Autodesk Inventor part; units mm, degrees
ref_plane "YZ Plane" through (0, 0, 0) normal (1, 0, 0) x (0, 1, 0)
ref_plane "XZ Plane" through (0, 0, 0) normal (0, 1, 0) x (-1, 0, 0)
ref_plane "XY Plane" through (0, 0, 0) normal (0, 0, 1) x (1, 0, 0)
sketch "Sketch1" plane through (0, 0, 0) normal (0, 0, 1) x (1, 0, 0)
  line L0 (0, 0) -> (33.25, 0)
  line L1 (33.25, 0) -> (33.25, 33.25)
  line L2 (33.25, 33.25) -> (0, 33.25)
  line L3 (0, 33.25) -> (0, 0)
  dimension "d0" = 33.25
  dimension "d1" = 33.25
extrude "Extrusion1" add sketch "Sketch1" along normal blind 30
sketch "Sketch2" plane through (0, 0, 30) normal (0, 0, 1) x (1, 0, 0)
  point P0 (0, 0)
sketch "Sketch3" plane through (0, 0, 30) normal (0, 0, 1) x (1, 0, 0)
  line L0 (3.25, 3.25) -> (30, 3.25)
  line L1 (30, 3.25) -> (30, 30)
  line L2 (30, 30) -> (3.25, 30)
  line L3 (3.25, 30) -> (3.25, 3.25)
  line L4 (33.25, 0) -> (33.25, 33.25)
  line L5 (0, 0) -> (33.25, 0)
  line L6 (33.25, 0) -> (33.25, 33.25)
  line L7 (33.25, 33.25) -> (0, 33.25)
  line L8 (0, 33.25) -> (0, 0)
  dimension "d4" = 26.75
  dimension "d5" = 26.75
extrude "Extrusion2" cut sketch "Sketch3" against normal blind 26.75 contours L3 L2 L1 L0
chamfer "Chamfer1" distance 1.875 angle 45 8 edges at (33.25, 33.25, 15) (33.25, 0, 15) (0, 33.25, 15) (0, 0, 15) (0, 16.625, 0) (16.625, 33.25, 0) (16.625, 0, 0) (33.25, 16.625, 0)
sketch "Sketch4" plane through (0, 0, 0) normal (0, 0, -1) x (-1, 0, 0)
  circle A0 centre (-16.625, 16.625) radius 4.625
  point P0 (0, 0)
  dimension "d11" = 9.25
properties part number "cuvette holder lid"
Could you check a few things on this model? Use its own coordinates, in mm. A direction names the side the tool comes from. Coordinates: 2 decimals unless noted, no trailing zeros. Write each loop counter-clockwise with the first axis right and the second up, starting at its lowest first coordinate (ties: lowest second). Pieces come first, ordered by that corner, then holes. Notation, with made-up numbers: (66.25, -19) - (108.25, -19) arc R20 cw to (108.25, 8) - close; hole circle Ø6 at (73.25, 59.5). An arc over 180 degrees is marked (long way). Put each result on its own line as item: value. Start each with the question number.
Q1. I want a section at A-A on z = 7.5. Write out the boundary of the cut face in (x, y) (3 decimals).
Q2. Thinking about a two-plate mould opening in X: for faces 3 (the flat face through (3.25, 17, 17)), 4 (the flat face through (16, 17, 0)), 5 (the flat face through (0.951, 32.326, 15.741)), which applies, pulls with the +X half, pulls with the -X half, needs draft (parallel to the pull), parting line crosses it, or undercut?
Q3. Please list where these lines run through material, in increasing order: L1, parallel to Y at x = 19, z = 4.25; L2, parallel to Z at x = 10.5, y = 16.
Q4. I want a section at B-B on x = 19.5. Write out the boundary of the cut face in (y, z) (3 decimals).
Q5. Which directions (+Z, -Z, +X, -X, +Y, -Y) give clear straight access to the entire face, cutting with the end or side of a thin tool? Please do faces 1 (the flat face through (2, 17, 30)), 2 (the flat face through (16, 17, 3.25)).
Q6. I'm going to push a flat-ended pin straight in: P1, Ø8, axis at x = 20.5, y = 12.5, coming from the +Z side. Where does the tip first touch, or does it pass through?
Checks:
1. outline: (0, 1.875) - (1.875, 0) - (31.375, 0) - (33.25, 1.875) - (33.25, 31.375) - (31.375, 33.25) - (1.875, 33.25) - (0, 31.375) - close; hole (3.25, 3.25) - (30, 3.25) - (30, 30) - (3.25, 30) - close
2. face 3: undercut
2. face 4: needs draft
2. face 5: pulls with the -X half
3. L1: 0 to 3.25, 30 to 33.25
3. L2: 0 to 3.25
4. outline: (0, 1.875) - (1.875, 0) - (31.375, 0) - (33.25, 1.875) - (33.25, 30) - (30, 30) - (30, 3.25) - (3.25, 3.25) - (3.25, 30) - (0, 30) - close
5. face 1: +Z, +X, -X, +Y, -Y
5. face 2: +Z
6. P1: z = 3.25
